from build123d import *

# Parameters (mm, degrees)
F0_W     = 15.24
F0_H     = 15.24
F1_DEPTH = 7.62
F3_D     = 2.2606
F3_DEPTH = 6.35
F3_TIP   = 0.6791527577
F6_D     = 2.2606
F6_DEPTH = 6.35
F6_TIP   = 0.6791527577
F7_D     = 2.2606
F7_DEPTH = 6.35
F7_TIP   = 0.6791527577


with BuildPart() as f1:
    # F0 (on Top) → F1 (new body, symmetric)
    with BuildSketch(Plane.XY):
        Rectangle(F0_W, F0_H)
    extrude(amount=F1_DEPTH, both=True)

    # F3
    with Locations(Plane.YZ.offset(7.62)):
        with Locations((0, 0)):
            Hole(F3_D / 2, depth=F3_DEPTH)
            with Locations((0, 0, -(F3_DEPTH + F3_TIP / 2))):  # 118° drill point
                Cone(0, F3_D / 2, F3_TIP, mode=Mode.SUBTRACT)

    # F6
    with Locations(Plane.XY.offset(7.62)):
        with Locations((0, 0)):
            Hole(F6_D / 2, depth=F6_DEPTH)
            with Locations((0, 0, -(F6_DEPTH + F6_TIP / 2))):  # 118° drill point
                Cone(0, F6_D / 2, F6_TIP, mode=Mode.SUBTRACT)

    # F7
    with Locations(Plane(origin=(0, 7.62, 0), x_dir=(-1, 0, 0), z_dir=(0, 1, 0))):
        with Locations((0, 0)):
            Hole(F7_D / 2, depth=F7_DEPTH)
            with Locations((0, 0, -(F7_DEPTH + F7_TIP / 2))):  # 118° drill point
                Cone(0, F7_D / 2, F7_TIP, mode=Mode.SUBTRACT)


solid = f1.part
For this review, take the finished solid that the model builds, in its own axes (mm). A direction names the side the tool comes from. Give positions to 0.01 mm unless a question says otherwise; leave off trailing zeros. Order: outer loops, then holes, each group sorted by start corner. A loop starts at its lowest first (then second) coordinate and runs counter-clockwise, first axis right, second up. Notation, with made-up numbers: (-27.75, 80.5) - (13.25, 80.5) arc R27 ccw to (13.25, 104.5) - close; hole circle Ø10 at (27, 49.25). An arc over 180 degrees is marked (long way). Answer as a JSON object with one key per item and string values. Group by question number.
Item 1: Clearance check with a flat-ended pin moving along its axis: pin 1 Ø1.5 at (x, z) = (1, 0) entering from +Y. State where the tip first meets the part, or that it passes through.
Item 2: Machinability: for faces 1 (the cylindrical face through (4.401, 0.245, -1.103)), 2 (the flat face through (2, 7.62, 0)), 3 (the flat face through (-7.62, 0, 0)), 4 (the cylindrical face through (0.245, -1.103, 4.401)), 5 (the cylindrical face through (-0.245, 4.401, -1.103)), which of the approach directions +Z, -Z, +X, -X, +Y, -Y give a long, thin tool a straight path to every point of the face, cutting with its end or side? Answer none if there is none.
Item 3: Take a section at A-A on z = 5. Give the boundary of the cut face in (x, y), and give its area (3 significant figures).
Item 4: Draft analysis for pull direction Y (two halves, no side actions). For faces 6 (the conical face through (0.71, -0.16, -0.12)), 7 (the flat face through (7.62, 2, 0)), 8 (the flat face through (0, -7.62, 0)), state which applies: pulls with the +Y half, pulls with the -Y half, needs draft (parallel to the pull), parting line crosses it, or undercut.
Item 5: Wall thickness on line 1 along X through (y, z) = (0, 3); line 2 along X through (y, z) = (4.75, -1): over which ranges is each line inside the solid? List them lowest first.
Reported:
{
 "1": {"pin 1": "y = 7.62"},
 "2": {"face 1": "+X", "face 2": "+Z, -Z, +X, -X, +Y", "face 3": "+Z, -Z, -X, +Y, -Y", "face 4": "+Z", "face 5": "+Y"},
 "3": {"outline": "(-7.62, -7.62) - (7.62, -7.62) - (7.62, 7.62) - (-7.62, 7.62) - close; hole circle Ø2.26 at (0, 0)", "area": "228 mm^2"},
 "4": {"face 6": "undercut", "face 7": "needs draft", "face 8": "pulls with the -Y half"},
 "5": {"line 1": "-7.62 to -1.13, 1.13 to 7.62", "line 2": "-7.62 to -0.53, 0.53 to 7.62"}
}
